Job drawing, mm, ordinate dimensions from the low corner. One solid piece. A direction names the side the tool comes from. Coordinates: 2 decimals unless noted, no trailing zeros. Order: outer loops, then holes, each group sorted by start corner. A loop starts at its lowest first (then second) coordinate and runs counter-clockwise, first axis right, second up. Notation, with made-up numbers: (32, 87) - (78, 87) arc R23 ccw to (78, 114) - close; hole circle Ø3 at (49.5, -12.75). An arc over 180 degrees is marked (long way). Use one line per item in the form item = value.
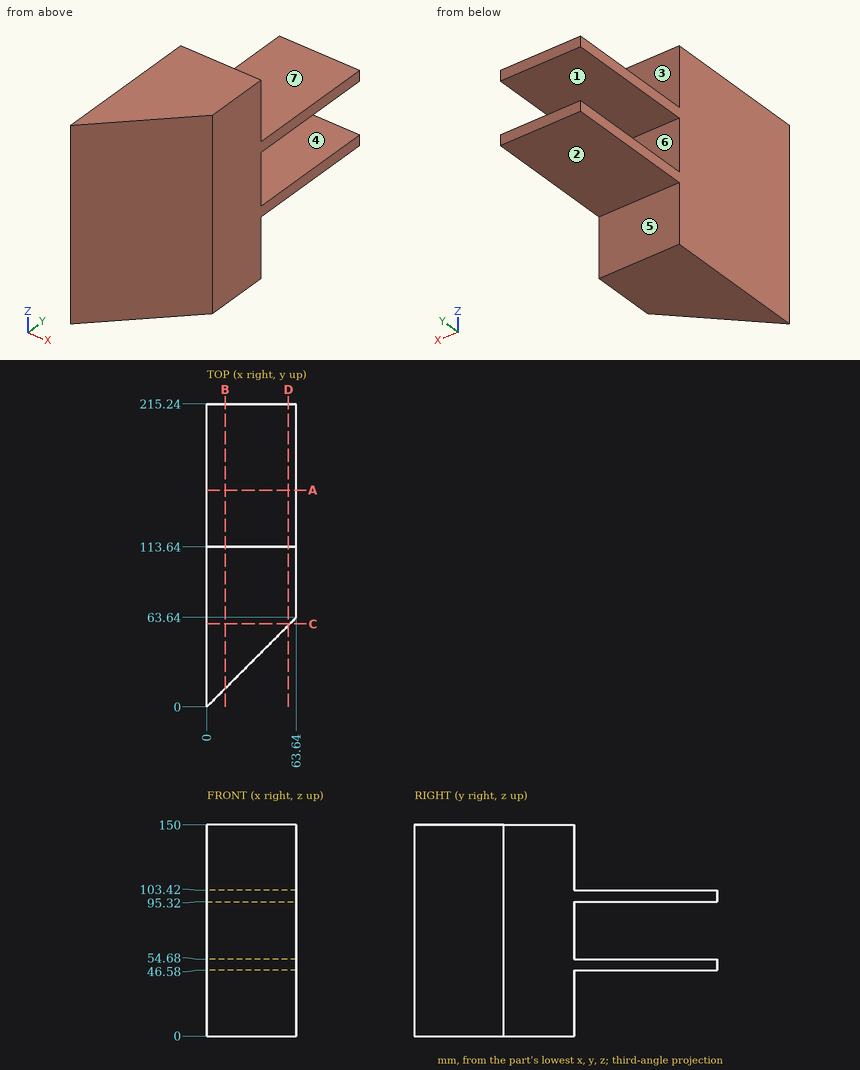
Item 1: Cut at C-C, the plane y = 59. Write the cut outline in (x, z), plus the area to 3 significant figures.
Derived:
outline = (0, 0) - (59, 0) - (59, 150) - (0, 150) - close
area = 8,850 mm²
Item 2: Cut at D-D, the plane x = 58. Write the cut outline in (y, z).
Derived:
outline = (58, 0) - (113.64, 0) - (113.64, 46.58) - (215.24, 46.58) - (215.24, 54.68) - (113.64, 54.68) - (113.64, 95.32) - (215.24, 95.32) - (215.24, 103.42) - (113.64, 103.42) - (113.64, 150) - (58, 150) - close
Item 3: Two-plate mould, pull along Z, no slides. Class the marked faces 4, 5, 6 and 7: +Z half, -Z half, draft (parallel to the pull), parting line (faces both ways), or undercut.
Derived:
face_4 = undercut
face_5 = draft
face_6 = undercut
face_7 = +Z half
Item 4: Drop flat-ended pins along their axis: pin 1 (1 mm diameter, centred on x = 7, z = 63.5, fed in from +Y); pin 2 (2 mm diameter, centred on x = 7, y = 152.5, fed in from +Z); pin 3 (19 mm diameter, centred on x = 32.5, y = 149.5, fed in from -Z). Give the stop position or say it passes through.
Derived:
pin_1 = 113.64
pin_2 = 103.42
pin_3 = 46.58
Item 5: Cut at A-A, the plane y = 154. Write the cut outline in (x, z).
Derived:
outline = (0, 46.58) - (63.64, 46.58) - (63.64, 54.68) - (0, 54.68) - close; (0, 95.32) - (63.64, 95.32) - (63.64, 103.42) - (0, 103.42) - close
Item 6: Drill centre lines: line 1 (Z direction, x = 14.5, y = 136.5); line 2 (X direction, y = 36.5, z = 85); line 3 (Y direction, x = 43.5, z = 65). Where is each one in solid material? Low to high. Write a range as [from, to].
Derived:
line_1 = [46.58, 54.68], [95.32, 103.42]
line_2 = [0, 36.5]
line_3 = [43.5, 113.64]
Item 7: 3-axis set-ups, long thin cutter, end or side, ignore diameter. For the marked faces 1, 2 and 3: which of +Z, -Z, +X, -X, +Y, -Y reach the whole face in a straight line?
Derived:
face_1 = +X, -X, +Y
face_2 = -Z, +X, -X, +Y
face_3 = +Z, +X, -X, +Y
Item 8: Cut at B-B, the plane x = 13. Write the cut outline in (y, z), plus the area to 3 significant figures.
Derived:
outline = (13, 0) - (113.64, 0) - (113.64, 46.58) - (215.24, 46.58) - (215.24, 54.68) - (113.64, 54.68) - (113.64, 95.32) - (215.24, 95.32) - (215.24, 103.42) - (113.64, 103.42) - (113.64, 150) - (13, 150) - close
area = 16,700 mm²
